Verification items for the finished model (mm, model axes). A direction names the side the tool comes from. Give positions to 0.01 mm unless a question says otherwise; leave off trailing zeros. Loops run counter-clockwise (first coordinate to the right, second up) from the corner with the lowest first, then second, coordinate; pieces in that order, holes last. Notation, with made-up numbers: (59, -20.5) - (87, -20.5) arc R26 ccw to (87, 2.5) - close; hole circle Ø8 at (46, -21.75). An arc over 180 degrees is marked (long way). Answer in a Markdown table with one row per item.
```python
from build123d import *

# Parameters (mm, degrees)
F0_R     = 36.5
F1_DEPTH = 25
F2_R     = 2
F3_R     = 34.5
F4_DEPTH = 17.2
F5_R     = 1
F6_DEPTH = 25


with BuildPart() as f1:
    # F0 (on Top) → F1 (new body)
    with BuildSketch(Plane.XY):
        Circle(F0_R)
    extrude(amount=F1_DEPTH)

    # F2
    f2_edges = [f1.edges().sort_by_distance(p)[0] for p in [
        (-36.5, 0, 0),
    ]]
    fillet(f2_edges, radius=F2_R)

    # F3 (on face) → F4 (cut)
    with BuildSketch(Plane.XY.offset(25)):
        Circle(F3_R)
    extrude(amount=-F4_DEPTH, mode=Mode.SUBTRACT)

    # F5 (on face) → F6 (cut)
    with BuildSketch(Plane.XY.offset(7.8)):
        Circle(F5_R)
    extrude(amount=-F6_DEPTH, mode=Mode.SUBTRACT)


solid = f1.part
```
Q1. Tool access check on faces 4 (the face through (0, -7, 7.8)), 5 (the face through (-22, -27, 25)). Record the directions out of +Z, -Z, +X, -X, +Y, -Y that give a thin tool (end or side, any length) a straight path to the whole face; none if there is none.
Completed:
| item | result |
|---|---|
| face 4 | +Z |
| face 5 | +Z, +X, -X, +Y, -Y |
Q2. Sectioned sample at A-A (y = 0). Record the cut outline in (x, z).
Completed:
| item | result |
|---|---|
| outline | (-36.5, 2) arc R2 ccw to (-34.5, 0) - (-1, 0) - (-1, 7.8) - (-34.5, 7.8) - (-34.5, 25) - (-36.5, 25) - close; (1, 0) - (34.5, 0) arc R2 ccw to (36.5, 2) - (36.5, 25) - (34.5, 25) - (34.5, 7.8) - (1, 7.8) - close |
Q3. Sectioned sample at C-C (z = 11.25). Record the cut outline in (x, y), and give its area (3 significant figures).
Completed:
| item | result |
|---|---|
| outline | circle Ø73 at (0, 0); hole circle Ø69 at (0, 0) |
| area | 446 mm^2 |
Q4. Thickness scan on line 1 (Y direction, x = 0, z = 16.5); line 2 (Y direction, x = 0, z = 5); line 3 (Z direction, x = 3, y = -9). Record the ranges inside material, lowest first.
Completed:
| item | result |
|---|---|
| line 1 | -36.5 to -34.5, 34.5 to 36.5 |
| line 2 | -36.5 to -1, 1 to 36.5 |
| line 3 | 0 to 7.8 |
Q5. Go/stop test with flat-tipped pins: P1, Ø10, axis at y = -16, z = 6.5, coming from the +X side; P2, Ø10, axis at x = -11, z = 21, coming from the -Y side; P3, Ø10, axis at x = -1, z = 17.5, coming from the -Y side. Record where each tip stops, or that it passes through.
Completed:
| item | result |
|---|---|
| P1 | x = 34.8 |
| P2 | y = -36 |
| P3 | y = -36.5 |
Q6. Draft check along Y on faces 1 (the face through (-7.912, -35.632, 13.339)), 2 (the face through (0, -7, 0)), 3 (the face through (32.907, 10.363, 16.52)). Enter one of: +Y half, -Y half, draft (parallel to the pull), parting line (faces both ways), or undercut.
Completed:
| item | result |
|---|---|
| face 1 | parting line |
| face 2 | draft |
| face 3 | undercut |
